The figure shows three views and two pictorial views of one solid part (mm, origin at its lowest corner). Answer the questions. Give positions to 0.01 mm unless a question says otherwise; leave off trailing zeros. Loops run counter-clockwise (first coordinate to the right, second up) from the corner with the lowest first, then second, coordinate; pieces in that order, holes last. Notation, with made-up numbers: (-31.5, -10.75) - (-24.5, -10.75) arc R34 cw to (-24.5, 21.25) - close; hole circle Ø5 at (58.25, 76). An arc over 180 degrees is marked (long way). Write item = value, one per line.
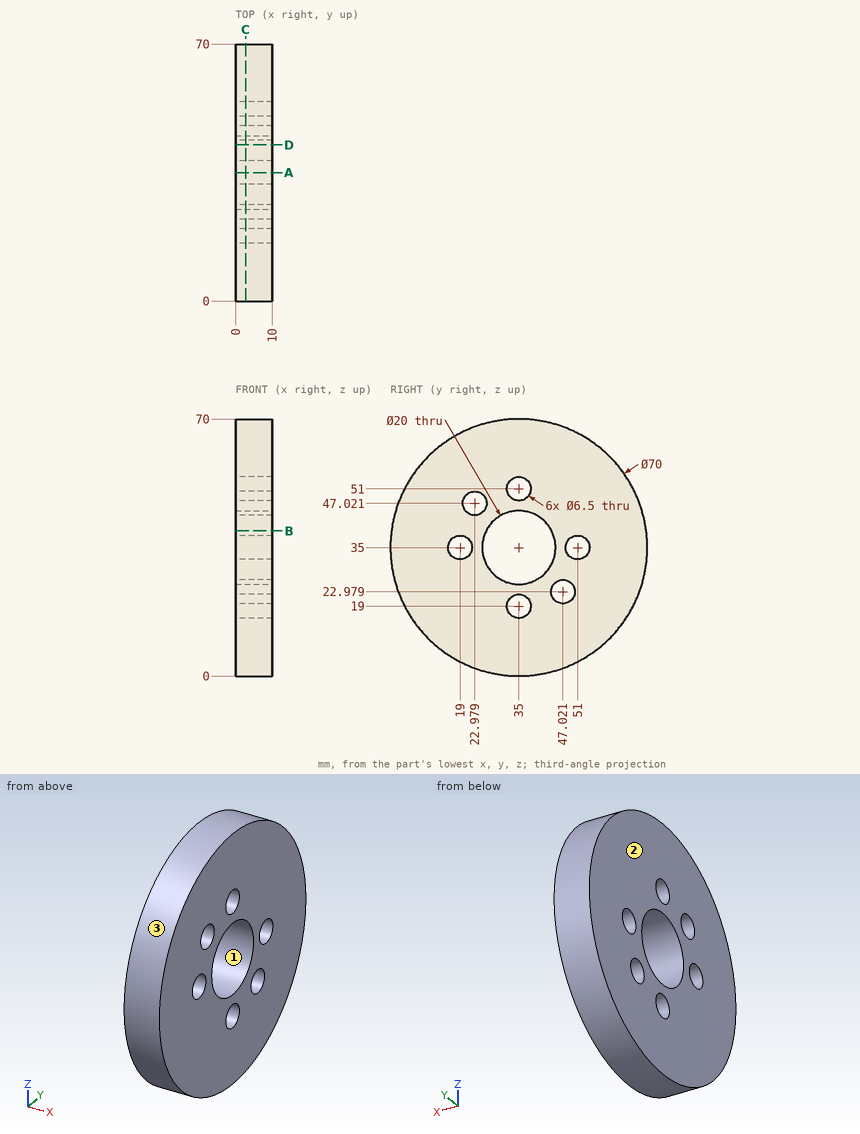
1) Find the intervals of material crossed by probe 1 along Y at (x, z) = (4, 35); probe 2 along Z at (x, y) = (8.5, 49); probe 3 along Z at (x, y) = (7.5, 32), in increasing order.
Output:
probe_1 = 0 to 15.75, 22.25 to 25, 45 to 47.75, 54.25 to 70
probe_2 = 2.92 to 20.4, 25.56 to 32.44, 37.56 to 67.08
probe_3 = 0.13 to 17.75, 20.25 to 25.46, 44.54 to 49.75, 52.25 to 69.87
2) A cutting plane is placed at A-A on y = 35. Determine the outline of the cut face in (x, z), then the cut area to 3 significant figures.
Output:
outline = (0, 0) - (10, 0) - (10, 15.75) - (0, 15.75) - close; (0, 22.25) - (10, 22.25) - (10, 25) - (0, 25) - close; (0, 45) - (10, 45) - (10, 47.75) - (0, 47.75) - close; (0, 54.25) - (10, 54.25) - (10, 70) - (0, 70) - close
area = 370 mm²
3) Each of these flat-tipped pins is pushed along its axis until it touches: P1, Ø1, axis at x = 7.5, z = 49, coming from the +Y side; P2, Ø6, axis at x = 1, y = 12, coming from the +Z side; P3, Ø6, axis at x = 7, z = 14.5, coming from the +Y side. Where does it stop, or does it pass through?
Output:
P1 = 67.29
P2 = 63.72
P3 = 65.31
4) The mould has two halves that part along Y. Classify the marked faces 1, 2 and 3: pulls with the +Y half, pulls with the -Y half, needs draft (parallel to the pull), parting line crosses it, or undercut.
Output:
face_1 = undercut
face_2 = needs draft
face_3 = parting line crosses it
5) A cutting plane is placed at D-D on y = 42.5. Determine the outline of the cut face in (x, z).
Output:
outline = (0, 0.81) - (10, 0.81) - (10, 28.39) - (0, 28.39) - close; (0, 41.61) - (10, 41.61) - (10, 69.19) - (0, 69.19) - close
6) A cutting plane is placed at C-C on x = 2.75. Determine the outline of the cut face in (y, z), then the cut area to 3 significant figures.
Output:
outline = circle Ø70 at (35, 35); hole circle Ø6.5 at (19, 35); hole circle Ø6.5 at (22.98, 47.02); hole circle Ø20 at (35, 35); hole circle Ø6.5 at (35, 19); hole circle Ø6.5 at (35, 51); hole circle Ø6.5 at (47.02, 22.98); hole circle Ø6.5 at (51, 35)
area = 3,340 mm²
7) A cutting plane is placed at B-B on z = 39.5. Determine the outline of the cut face in (x, y), then the cut area to 3 significant figures.
Output:
outline = (0, 0.29) - (10, 0.29) - (10, 26.07) - (0, 26.07) - close; (0, 43.93) - (10, 43.93) - (10, 69.71) - (0, 69.71) - close
area = 516 mm²
